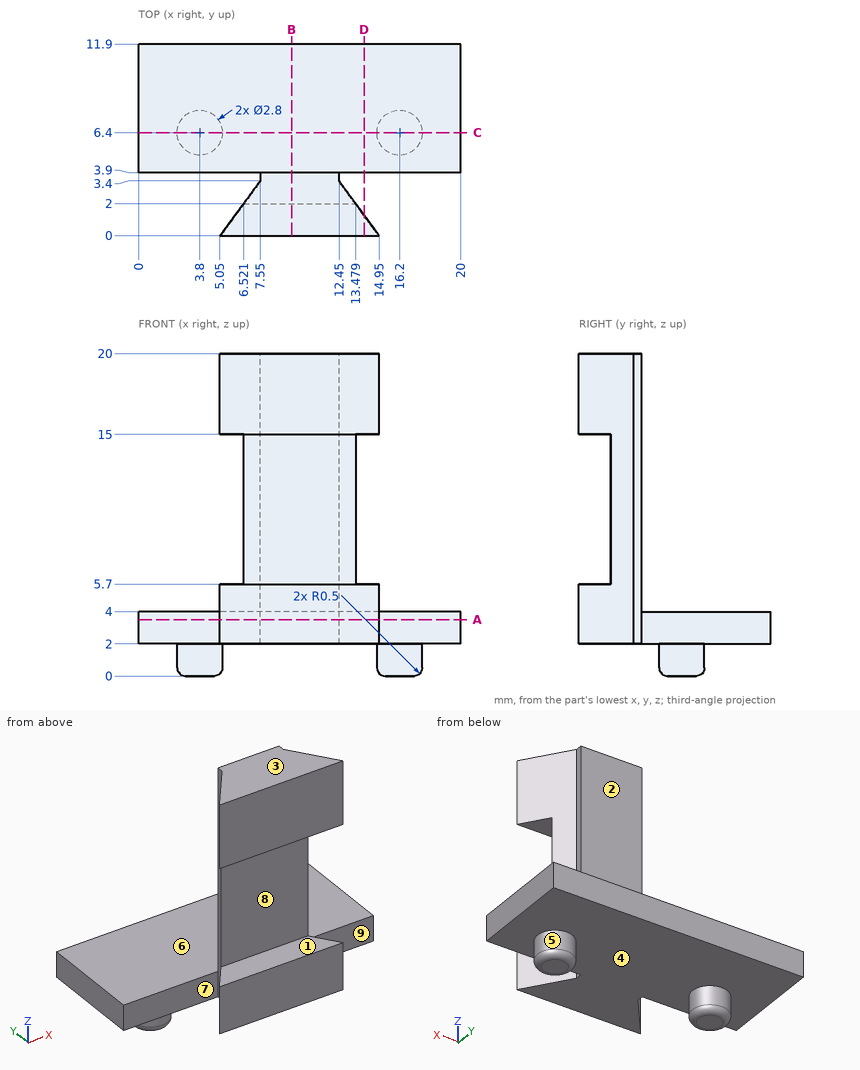
Answer from the drawing. Dimensions are ordinates in mm from the lowest x, y and z of the part. A direction names the side the tool comes from. Coordinates: 2 decimals unless noted, no trailing zeros. Write each loop counter-clockwise with the first axis right and the second up, starting at its lowest first coordinate (ties: lowest second). Pieces come first, ordered by that corner, then holes. Notation, with made-up numbers: (57.25, 46.5) - (86.25, 46.5) arc R22 cw to (86.25, 64.5) - close; hole circle Ø1 at (-20.75, 13). An arc over 180 degrees is marked (long way). One line per question, with ' | ' between items.
Q1. Find section D-D, the plane x = 14. Write down the section's boundary in (y, z).
Result set:
outline: (0, 2) - (1.29, 2) - (1.29, 5.7) - (0, 5.7) - close; (0, 15) - (1.29, 15) - (1.29, 20) - (0, 20) - close; (3.9, 2) - (11.9, 2) - (11.9, 4) - (3.9, 4) - close
Q2. Each of these flat-tipped pins is pushed along its axis until it touches: P1, Ø3.5, axis at x = 10, z = 9, coming from the -Y side; P2, Ø0.6, axis at y = 3.5, z = 11.5, coming from the +X side; P3, Ø1.6, axis at x = 9, y = 1, coming from the -Z side. Where does it stop, or does it pass through?
Result set:
P1: y = 2 | P2: x = 12.6 | P3: z = 2
Q3. Consider L1, parallel to Z at x = 5, y = 7.5; L2, parallel to X at y = 3.75, z = 12.75; L3, parallel to Y at x = 12, z = 12.25. Determine where each line is inside the solid, lowest interval first. Write a range as [from, to].
Result set:
L1: [2, 4] | L2: [7.55, 12.45] | L3: [2, 3.9]
Q4. Find section C-C, the plane y = 6.4. Write down the section's boundary in (x, z).
Result set:
outline: (0, 2) - (2.4, 2) - (2.4, 0.5) arc R0.5 ccw to (2.9, 0) - (4.7, 0) arc R0.5 ccw to (5.2, 0.5) - (5.2, 2) - (14.8, 2) - (14.8, 0.5) arc R0.5 ccw to (15.3, 0) - (17.1, 0) arc R0.5 ccw to (17.6, 0.5) - (17.6, 2) - (20, 2) - (20, 4) - (0, 4) - close
Q5. For the marked faces 5, 6, 7, 8 and 9, determine the directions among +Z, -Z, +X, -X, +Y, -Y from which every point of the face is accessible in a straight line to the end or side of a thin tool.
Result set:
face 5: -Z | face 6: +Z, +X, -X, +Y | face 7: +Z, -Z, -X | face 8: +X, -X, -Y | face 9: +Z, -Z, +X
Q6. Find section A-A, the plane z = 3.5. Write down the section's boundary in (x, y), plus the area to 3 significant figures.
Result set:
outline: (0, 3.9) - (7.55, 3.9) - (7.55, 3.4) - (5.05, 0) - (14.95, 0) - (12.45, 3.4) - (12.45, 3.9) - (20, 3.9) - (20, 11.9) - (0, 11.9) - close | area: 188 mm^2
Q7. Determine the mould class of the marked faces 1, 2, 3 and 4 for opening direction Z: +Z half, -Z half, draft (parallel to the pull), parting line (faces both ways), or undercut.
Result set:
face 1: undercut | face 2: draft | face 3: +Z half | face 4: -Z half
Q8. Find section B-B, the plane x = 9.5. Write down the section's boundary in (y, z).
Result set:
outline: (0, 2) - (11.9, 2) - (11.9, 4) - (3.9, 4) - (3.9, 20) - (0, 20) - (0, 15) - (2, 15) - (2, 5.7) - (0, 5.7) - close
